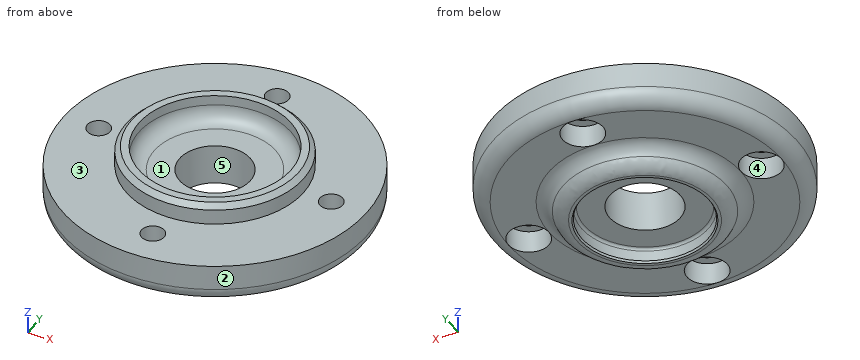
Autodesk Inventor part; units mm, degrees
ref_plane "YZ Plane" through (0, 0, 0) normal (1, 0, 0) x (0, 1, 0)
ref_plane "XZ Plane" through (0, 0, 0) normal (0, 1, 0) x (-1, 0, 0)
ref_plane "XY Plane" through (0, 0, 0) normal (0, 0, 1) x (1, 0, 0)
sketch "스케치1" plane through (0, 0, 0) normal (0, 0, 1) x (1, 0, 0)
  circle A0 centre (0, 0) radius 30
  dimension "d0" = 60
extrude "돌출1" add sketch "스케치1" along normal blind 8
sketch "스케치2" plane through (0, 0, 8) normal (0, 0, 1) x (1, 0, 0)
  circle A0 centre (0, 0) radius 17.5
  dimension "d3" = 35
extrude "돌출2" add sketch "스케치2" along normal blind 4
sketch "스케치3" plane through (0, 0, 0) normal (0, 0, -1) x (-1, 0, 0)
  circle A0 centre (0, 0) radius 16
  dimension "d6" = 32
extrude "돌출3" add sketch "스케치3" along normal blind 4
sketch "스케치4" plane through (0, 0, 12) normal (0, 0, 1) x (1, 0, 0)
  circle A0 centre (0, 0) radius 15
  dimension "d9" = 30
extrude "돌출4" cut sketch "스케치4" against normal blind 5
sketch "스케치5" plane through (0, 0, 7) normal (0, 0, 1) x (1, 0, 0)
  circle A0 centre (0, 0) radius 7
  dimension "d12" = 14
extrude "돌출5" cut sketch "스케치5" against normal blind 8
sketch "스케치6" plane through (0, 0, -1) normal (0, 0, 1) x (1, 0, 0)
  circle A0 centre (0, 0) radius 12.5
  dimension "d15" = 25
extrude "돌출6" cut sketch "스케치6" against normal up to next
sketch "스케치7" plane through (0, 0, 0) normal (0, 0, -1) x (-1, 0, 0)
  circle A0 centre (0, 23) radius 2.25
  point P0 (0, 0)
  dimension "d18" = 4.5
  dimension "d19" = 23
hole "구멍1" at (0, 23, 0) direction (0, 0, 1) diameter 4.5 end through all counterbore diameter 8 counterbore depth 4.4
pattern_circular "원형 패턴1" count 4 over 360 about axis through (0, 0, 0) along (0, 0, 1) of "구멍1"
chamfer "모따기1" distance 0.4 angle 30 1 edges at (-12.5, 0, -4) measured on face at (12.4595, -1.0058, -3)
fillet "모깎기1" radius 0.5 1 edges at (-12.5, 0, -1)
chamfer "모따기2" distance 1 angle 45 1 edges at (-17.5, 0, 12)
fillet "모깎기2" radius 3 4 edges at (-30, 0, 0) (16, 0, 0) (16, 0, -4) (-15, 0, 7)
properties part number "2강"
Work out the finished part from the listing and answer in its coordinate system (mm). Face numbers are marked on the shaded views. A direction names the side the tool comes from. Give positions to 0.01 mm unless a question says otherwise; leave off trailing zeros. Order: outer loops, then holes, each group sorted by start corner. A loop starts at its lowest first (then second) coordinate and runs counter-clockwise, first axis right, second up.
1. Section B-B, the plane x = 0 is taken. Give the number of separate pieces and of enclosed holes in the cut face, and give its area (3 significant figures).
Result sheet:
separate pieces: 4
enclosed holes: 0
area: 309 mm2
2. For the marked faces 4 and 5, determine the directions among +Z, -Z, +X, -X, +Y, -Y from which every point of the face is accessible in a straight line to the end or side of a thin tool.
Result sheet:
face 4: -Z
face 5: +Z, -Z
3. Each of these flat-tipped pins is pushed along its axis until it touches: P1, Ø5, axis at y = -15, z = 1, coming from the +X side; P2, Ø6.5, axis at x = 0, y = -22.5, coming from the -Z side; P3, Ø5, axis at x = -23, y = 0, coming from the +Z side. Where does it stop, or does it pass through?
Result sheet:
P1: stops at x = 27.01
P2: stops at z = 4.4
P3: stops at z = 8
4. Straight lines are drawn through the part: L1, parallel to Z at x = -13.5, y = 22.5; L2, parallel to Y at x = 0, z = 11.15; L3, parallel to X at y = 11.5, z = -2. For each, find the intervals that lie inside material, in ascending order.
Result sheet:
L1: z = 0 to 8
L2: y = -17.35 to -15, 15 to 17.35
L3: x = -11.37 to -4.9, 4.9 to 11.37
5. Section A-A, the plane z = 1.25 is taken. Determine the outline of the cut face in (x, y).
Result sheet:
outline: circle Ø58.87 at (0, 0); hole circle Ø8 at (-23, 0); hole circle Ø14 at (0, 0); hole circle Ø8 at (0, -23); hole circle Ø8 at (0, 23); hole circle Ø8 at (23, 0)
6. The mould has two halves that part along X. Classify the marked faces 1, 2 and 3: released by +X, released by -X, zero draft, split by the parting line, or undercut.
Result sheet:
face 1: undercut
face 2: split by the parting line
face 3: zero draft
